from build123d import *

# Parameters (mm, degrees)
SKETCH1_R           = 7.3
SKETCH1_R_2         = 6.6
BOSS_EXTRUDE1_DEPTH = 11.3
BOSS_EXTRUDE2_START = -2
SKETCH1_3_R         = 8.5
SKETCH1_3_R_2       = 6.6
BOSS_EXTRUDE2_DEPTH = 2
BOSS_EXTRUDE3_START = 11.3
SKETCH1_4_R         = 8.5
SKETCH1_4_R_2       = 6.6
BOSS_EXTRUDE3_DEPTH = 2
FILLET1_R           = 1.5
FILLET2_R           = 0.2
CUT_EXTRUDE1_START  = 13.3
SKETCH1_6_W         = 18
SKETCH1_6_H         = 3
CUT_EXTRUDE1_DEPTH  = 8
CUT_EXTRUDE3_START  = 13.3
SKETCH3_W           = 3
SKETCH3_H           = 22.651300202
CUT_EXTRUDE3_DEPTH  = 8


with BuildPart() as part:
    # Sketch1 → Boss-Extrude1 (new body)
    with BuildSketch(Plane(origin=(0, 0, 0), x_dir=(1, 0, 0), z_dir=(0, 1, 0))):
        with Locations(Location((0, 0, 0), (0, 0, 270))):
            Circle(SKETCH1_R)
        with Locations(Location((0, 0, 0), (0, 0, 270))):
            Circle(SKETCH1_R_2, mode=Mode.SUBTRACT)
    extrude(amount=BOSS_EXTRUDE1_DEPTH)

    # Sketch1<3> → Boss-Extrude2 (add)
    with BuildSketch(Plane(origin=(0, 0, 0), x_dir=(1, 0, 0), z_dir=(0, 1, 0)).offset(BOSS_EXTRUDE2_START)):
        with Locations(Location((0, 0, 0), (0, 0, 270))):
            Circle(SKETCH1_3_R)
        with Locations(Location((0, 0, 0), (0, 0, 270))):
            Circle(SKETCH1_3_R_2, mode=Mode.SUBTRACT)
    extrude(amount=BOSS_EXTRUDE2_DEPTH)

    # Sketch1<4> → Boss-Extrude3 (add)
    with BuildSketch(Plane(origin=(0, 0, 0), x_dir=(1, 0, 0), z_dir=(0, 1, 0)).offset(BOSS_EXTRUDE3_START)):
        with Locations(Location((0, 0, 0), (0, 0, 270))):
            Circle(SKETCH1_4_R)
        with Locations(Location((0, 0, 0), (0, 0, 270))):
            Circle(SKETCH1_4_R_2, mode=Mode.SUBTRACT)
    extrude(amount=BOSS_EXTRUDE3_DEPTH)

    # Fillet1
    fillet1_edges = [part.edges().sort_by_distance(p)[0] for p in [
        (0, 13.3, -8.5),
    ]]
    fillet(fillet1_edges, radius=FILLET1_R)

    # Fillet2
    fillet2_edges = [part.edges().sort_by_distance(p)[0] for p in [
        (0, 11.3, -8.5),
    ]]
    fillet(fillet2_edges, radius=FILLET2_R)

    # Sketch1<6> → Cut-Extrude1 (cut)
    with BuildSketch(Plane(origin=(0, 0, 0), x_dir=(1, 0, 0), z_dir=(0, 1, 0)).offset(CUT_EXTRUDE1_START)):
        Rectangle(SKETCH1_6_W, SKETCH1_6_H)
    extrude(amount=-CUT_EXTRUDE1_DEPTH, mode=Mode.SUBTRACT)

    # Sketch3 → Cut-Extrude3 (cut)
    with BuildSketch(Plane(origin=(0, 0, 0), x_dir=(1, 0, 0), z_dir=(0, 1, 0)).offset(CUT_EXTRUDE3_START)):
        Rectangle(SKETCH3_W, SKETCH3_H)
    extrude(amount=-CUT_EXTRUDE3_DEPTH, mode=Mode.SUBTRACT)


solid = part.part
Geometry: final body of the model. Coordinates: model frame, mm. A direction names the side the tool comes from. Round coordinates to 2 decimals unless told otherwise and drop trailing zeros. Loops run counter-clockwise (first coordinate to the right, second up) from the corner with the lowest first, then second, coordinate; pieces in that order, holes last. Notation, with made-up numbers: M 43,37.5 L 73,37.5 A17 cw 73,46.5 Z; hole C -13,71.5 d2. An arc over 180 degrees is marked long. Put each result on its own line as item: value. Start each with the question number.
(1) Section query C-C (y = 6). Return loops of the section in (x, z).
(2) Material intervals for line 1 along X through (y, z) = (1.75, 0); line 2 along Y through (x, z) = (0.25, 7.5); line 3 along Z through (x, y) = (7, 12.5), sorted ascending. Write a range as [from, to].
(3) Section query B-B (x = 0). Return loops of the section in (y, z).
(4) Section query D-D (y = 2.25). Return loops of the section in (x, z), then the cut area to 3 significant figures.
(5) Contact query for flat-ended pins moving along their axis: pin 1 Ø1 at (x, z) = (0.5, -7) entering from +Y; pin 2 Ø6 at (x, y) = (0.5, 9.5) entering from +Z; pin 3 Ø2 at (y, z) = (9.5, -7.5) entering from +X. Output: stop coordinate, or through.
(6) Section query A-A (z = 0). Return loops of the section in (x, y), then the cut area to 3 significant figures.
(7) Draft query along X for faces 4 (the face through (1.5, 10.24, -6.95)), 5 (the face through (8.428, -1.014, -1.107)), 6 (the face through (-5.96, 11.65, -6.06)). Return one class per face: +X half, -X half, draft (parallel to the pull), parting line (faces both ways), or undercut.
(8) Set-up query: faces 1 (the face through (7, 0, -3)), 2 (the face through (5.3, 11.3, 5.3)), 3 (the face through (-1.5, 10.24, -6.95)). Return all of +Z, -Z, +X, -X, +Y, -Y with unobstructed straight access to the full face (end or side cutting, diameter ignored); none if empty.
Findings below:
1. outline: M -7.14,-1.5 A7.3 ccw -1.5,-7.14 L -1.5,-6.43 A6.6 cw -6.43,-1.5 Z; M -7.14,1.5 L -6.43,1.5 A6.6 cw -1.5,6.43 L -1.5,7.14 A7.3 ccw Z; M 1.5,-7.14 A7.3 ccw 7.14,-1.5 L 6.43,-1.5 A6.6 cw 1.5,-6.43 Z; M 1.5,6.43 A6.6 cw 6.43,1.5 L 7.14,1.5 A7.3 ccw 1.5,7.14 Z
2. line 1: x = [-7.3, -6.6], [6.6, 7.3]
2. line 2: y = [-2, 0]
2. line 3: z = [-4.51, -1.5], [1.5, 4.51]
3. outline: M -2,-8.5 L 0,-8.5 L 0,-7.3 L 5.3,-7.3 L 5.3,-6.6 L -2,-6.6 Z; M -2,6.6 L 5.3,6.6 L 5.3,7.3 L 0,7.3 L 0,8.5 L -2,8.5 Z
4. outline: C 0,0 d14.6; hole C 0,0 d13.2
4. area: 30.6 mm2
5. pin 1: stops at y = 5.3
5. pin 2: stops at z = 8.37
5. pin 3: stops at x = 3.32
6. outline: M -8.5,-2 L -6.6,-2 L -6.6,5.3 L -7.3,5.3 L -7.3,0 L -8.5,0 Z; M 6.6,-2 L 8.5,-2 L 8.5,0 L 7.3,0 L 7.3,5.3 L 6.6,5.3 Z
6. area: 15.0 mm2
7. face 4: undercut
7. face 5: parting line
7. face 6: -X half
8. face 1: none
8. face 2: +Z, +X
8. face 3: +Z, -Z, +Y
